Input: dimensioned drawing with shaded views. Units: mm. Origin: part minimum x, y, z. A direction names the side the tool comes from. Round coordinates to 2 decimals unless told otherwise and drop trailing zeros. Loops run counter-clockwise (first coordinate to the right, second up) from the corner with the lowest first, then second, coordinate; pieces in that order, holes last. Notation, with made-up numbers: (6, 17) - (17, 17) arc R17 cw to (17, 21) - close; hole circle Ø8 at (37, -28.75). An arc over 180 degrees is marked (long way). One line per question, with ' | ' between items. Start each with the question number.
1. Cut plane A-A (x = 5). Return loops of the section in (y, z).
2. Cut plane B-B (y = 26.75). Return loops of the section in (x, z).
3. Cut plane D-D (z = 16.5). Return loops of the section in (x, y).
4. Cut plane C-C (z = 7.5). Return loops of the section in (x, y), then the cut area to 3 significant figures.
5. Ray query, line 1 (X direction, y = 29.6, z = 7.5); line 2 (Y direction, x = 20, z = 14.5); line 3 (Y direction, x = 37, z = 9.75). Return the intervals inside material, ascending.
6. Pin query (flat end, axial travel): pin 1 (5 mm diameter, centred on y = 14.5, z = 13.5, fed in from +X); pin 2 (13 mm diameter, centred on x = 19, y = 17.5, fed in from -Z); pin 3 (3 mm diameter, centred on x = 32.5, z = 7.5, fed in from -Y); pin 4 (10 mm diameter, centred on y = 9.5, z = 11.5, fed in from -X). Return the tip coordinate at first contact, or that it passes through.
7. Mould query, pull axis Y, two halves, no side actions, for the marked faces 1, 2 and 3. Classes: pulls with the +Y half, pulls with the -Y half, needs draft (parallel to the pull), parting line crosses it, or undercut.
8. Access query for the marked faces 4, 5, 6 and 7. Directions: +Z, -Z, +X, -X, +Y, -Y. A direction counts if a zero-diameter tool reaches every point of the face in a straight line with its end or side. Return the directions, or none.
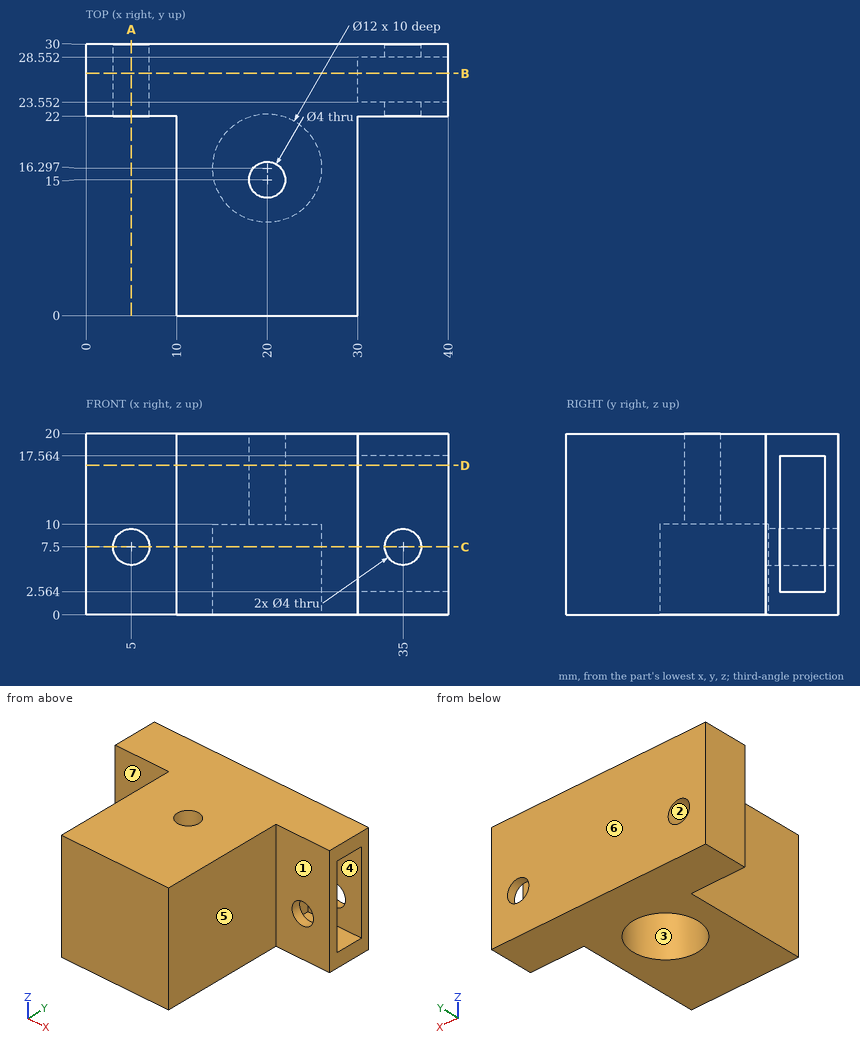
Answers follow:
1) outline: (22, 0) - (30, 0) - (30, 5.5) - (22, 5.5) - close; (22, 9.5) - (30, 9.5) - (30, 20) - (22, 20) - close
2) outline: (0, 0) - (40, 0) - (40, 2.56) - (30, 2.56) - (30, 17.56) - (40, 17.56) - (40, 20) - (0, 20) - close; hole circle Ø4 at (5, 7.5)
3) outline: (0, 22) - (10, 22) - (10, 0) - (30, 0) - (30, 22) - (40, 22) - (40, 23.55) - (30, 23.55) - (30, 28.55) - (40, 28.55) - (40, 30) - (0, 30) - close; hole circle Ø4 at (20, 15)
4) outline: (0, 22) - (3, 22) - (3, 30) - (0, 30) - close; (7, 22) - (10, 22) - (10, 0) - (30, 0) - (30, 22) - (33, 22) - (33, 23.55) - (30, 23.55) - (30, 28.55) - (33, 28.55) - (33, 30) - (7, 30) - close; (37, 22) - (40, 22) - (40, 23.55) - (37, 23.55) - close; (37, 28.55) - (40, 28.55) - (40, 30) - (37, 30) - close; hole circle Ø12 at (20, 16.3) | area: 553 mm2
5) line 1: x = 0 to 3, 7 to 33, 37 to 40 | line 2: y = 0 to 13, 17 to 30 | line 3: y = 22 to 23.55, 28.55 to 30
6) pin 1: stops at x = 30 | pin 2: stops at z = 0 | pin 3: stops at y = 22 | pin 4: stops at x = 10
7) face 1: pulls with the -Y half | face 2: needs draft | face 3: undercut
8) face 4: +X | face 5: +Z, -Z, +X, -Y | face 6: +Z, -Z, +X, -X, +Y | face 7: +Z, -Z, -X, -Y
